```python
from build123d import *

# Parameters (mm, degrees)
BOSS_EXTRUDE1_DEPTH = 20
BOSS_EXTRUDE2_START = 20
SKETCH1_3_R         = 10
BOSS_EXTRUDE2_DEPTH = 50
SKETCH2_R           = 15
BOSS_EXTRUDE3_DEPTH = 30


with BuildPart() as part:
    # Sketch1 → Boss-Extrude1 (new body)
    with BuildSketch(Plane.XY):
        with BuildLine():
            Line((-75, -335.522292415), (75, -335.522292415))
            Line((75, -335.522292415), (75, -85.522292415))
            ThreePointArc((75, -85.522292415), (108.166019919, -35.201912374), (110.9687456, 25))
            Line((110.9687456, 25), (-110.9687456, 25))
            ThreePointArc((-110.9687456, 25), (-108.166019919, -35.201912374), (-75, -85.522292415))
            Line((-75, -85.522292415), (-75, -335.522292415))
        make_face()
    extrude(amount=BOSS_EXTRUDE1_DEPTH)

    # Sketch1<3> → Boss-Extrude2 (add)
    with BuildSketch(Plane.XY.offset(BOSS_EXTRUDE2_START)):
        Circle(SKETCH1_3_R)
    extrude(amount=BOSS_EXTRUDE2_DEPTH)

    # Sketch2 → Boss-Extrude3 (add)
    with BuildSketch(Plane.XY.offset(20)):
        with Locations((0, -300)):
            Circle(SKETCH2_R)
    extrude(amount=BOSS_EXTRUDE3_DEPTH)


solid = part.part
```
Verification items for the finished model (mm, model axes). A direction names the side the tool comes from. Round coordinates to 2 decimals unless told otherwise and drop trailing zeros. Loops run counter-clockwise (first coordinate to the right, second up) from the corner with the lowest first, then second, coordinate; pieces in that order, holes last. Notation, with made-up numbers: (36.5, 18.5) -> (62.5, 18.5) arc R19 cw to (62.5, 36.5) -> close; hole circle Ø1 at (81.5, 71). An arc over 180 degrees is marked (long way). Answer as a JSON object with one key per item and string values.
Q1. Access from +Z, -Z, +X, -X, +Y, -Y to the whole of each face (thin tool, end or side, straight path). Record for faces 4 (the flat face through (0, -300, 50)), 5 (the cylindrical face through (-1.953, -285.128, 34.79)), 6 (the flat face through (75, -212, 10)).
Data:
{"face 4": "+Z, +X, -X, -Y", "face 5": "+Z", "face 6": "+Z, -Z, +X, -Y"}
Q2. Section check B-B (y = -300). Record the boundary of the cut face in (x, z), then the cut area to 3 significant figures.
Data:
{"outline": "(-75, 0) -> (75, 0) -> (75, 20) -> (15, 20) -> (15, 50) -> (-15, 50) -> (-15, 20) -> (-75, 20) -> close", "area": "3,900 mm2"}
Q3. Section check D-D (y = 0). Record the boundary of the cut face in (x, z).
Data:
{"outline": "(-113.75, 0) -> (113.75, 0) -> (113.75, 20) -> (10, 20) -> (10, 70) -> (-10, 70) -> (-10, 20) -> (-113.75, 20) -> close"}
Q4. Section check C-C (z = 26). Record the boundary of the cut face in (x, y), then the cut area to 3 significant figures.
Data:
{"outline": "circle Ø30 at (0, -300); circle Ø20 at (0, 0)", "area": "1,020 mm2"}
Q5. Draft check along Y on faces 1 (the flat face through (0, 0, 70)), 2 (the cylindrical face through (-2.17, -9.76, 44.65)), 3 (the flat face through (2, 25, 10)). Enter one of: pulls with the +Y half, pulls with the -Y half, needs draft (parallel to the pull), parting line crosses it, or undercut.
Data:
{"face 1": "needs draft", "face 2": "undercut", "face 3": "pulls with the +Y half"}
Q6. Go/stop test with flat-tipped pins: P1, Ø8, axis at y = -15, z = 28, coming from the +X side; P2, Ø4, axis at y = -81.5, z = 9, coming from the +X side; P3, Ø1.5, axis at x = 11, z = 34.5, coming from the -Y side; P4, Ø6, axis at y = -279, z = 12.5, coming from the +X side. Record where each tip stops, or that it passes through.
Data:
{"P1": "passes through", "P2": "stops at x = 81.36", "P3": "stops at y = -310.95", "P4": "stops at x = 75"}
Q7. Section check A-A (x = 0). Record the boundary of the cut face in (y, z), then the cut area to 3 significant figures.
Data:
{"outline": "(-335.52, 0) -> (25, 0) -> (25, 20) -> (10, 20) -> (10, 70) -> (-10, 70) -> (-10, 20) -> (-285, 20) -> (-285, 50) -> (-315, 50) -> (-315, 20) -> (-335.52, 20) -> close", "area": "9,110 mm2"}
Q8. Scan lines: line 1 (Y direction, x = -0.5, z = 38.5); line 2 (Z direction, x = 34, y = -193.5); line 3 (X direction, y = -224, z = 14). Record each from-to range of solid material in increasing order. Write a range as from..to.
Data:
{"line 1": "y = -314.99..-285.01, -9.99..9.99", "line 2": "z = 0..20", "line 3": "x = -75..75"}
